Here's how the part is built. I have some questions about the finished solid (model axes, mm). Face numbers are marked on the shaded views. A direction names the side the tool comes from. Round coordinates to 2 decimals unless told otherwise and drop trailing zeros. Loops run counter-clockwise (first coordinate to the right, second up) from the corner with the lowest first, then second, coordinate; pieces in that order, holes last. Notation, with made-up numbers: M 37,31 L 70,31 A18 ccw 70,48 Z; hole C -5.5,79 d3. An arc over 180 degrees is marked long. Use a Markdown table: item, result.
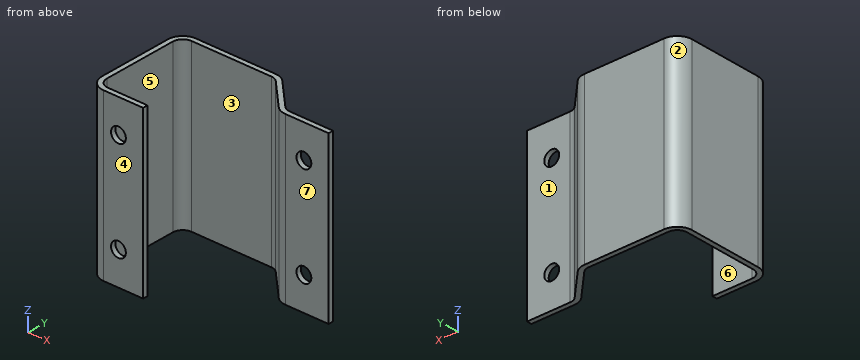
```python
from build123d import *

# Parameters (mm, degrees)
SKETCH1_W                    = 15
SKETCH1_H                    = 50
SKETCH1_R                    = 2.25
BASE_FLANGE1_DEPTH           = 1.5
EDGE_FLANGE1_STRIP_W         = 12
EDGE_FLANGE1_STRIP_H         = 1.5
EDGE_FLANGE1_STRIP_CUT_DEPTH = 50
EDGE_FLANGE1_DEPTH           = 50
EDGE_FLANGE2_STRIP_W         = 12
EDGE_FLANGE2_STRIP_H         = 1.5
EDGE_FLANGE2_STRIP_CUT_DEPTH = 50
EDGE_FLANGE2_DEPTH           = 50
EDGE_FLANGE3_STRIP_CUT_DEPTH = 50
EDGE_FLANGE3_DEPTH           = 50
EDGE_FLANGE4_STRIP_CUT_DEPTH = 50
EDGE_FLANGE4_DEPTH           = 50
SKETCH19_R                   = 2.25
CUT_EXTRUDE1_DEPTH           = 57.865713883


# Sheet-metal steps are written as plain solids
with BuildPart() as part:
    # Sketch1 → Base-Flange1 (new body)
    with BuildSketch(Plane(origin=(0, 0, 0), x_dir=(1, 0, 0), z_dir=(0, 1, 0))):
        Rectangle(SKETCH1_W, SKETCH1_H)
        with Locations(Location((0, 15, 0), (0, 0, 270))):
            Circle(SKETCH1_R, mode=Mode.SUBTRACT)
        with Locations(Location((0, -15, 0), (0, 0, 270))):
            Circle(SKETCH1_R, mode=Mode.SUBTRACT)
    extrude(amount=BASE_FLANGE1_DEPTH)

    # Edge-Flange1 strip (across the edge) → Edge-Flange1 strip cut (cut)
    with BuildSketch(Plane(origin=(-7.5, 1.5, -25), x_dir=(1, 0, 0), z_dir=(0, 0, 1))):
        with Locations((-3, -0.75)):
            Rectangle(EDGE_FLANGE1_STRIP_W, EDGE_FLANGE1_STRIP_H)
    extrude(amount=EDGE_FLANGE1_STRIP_CUT_DEPTH, mode=Mode.SUBTRACT)

    # Edge-Flange1 section (across the edge) → Edge-Flange1 (add)
    with BuildSketch(Plane(origin=(-7.5, 1.5, -25), x_dir=(1, 0, 0), z_dir=(0, 0, 1))):
        with BuildLine():
            Line((-1.5, 3), (-1.5, 28.5))
            Line((-1.5, 28.5), (0, 28.5))
            Line((0, 28.5), (0, 3))
            ThreePointArc((0, 3), (0.878679656, 0.878679656), (3, 0))
            Line((3, 0), (3, -1.5))
            ThreePointArc((3, -1.5), (-0.181980515, -0.181980515), (-1.5, 3))
        make_face()
    extrude(amount=EDGE_FLANGE1_DEPTH)

    # Edge-Flange2 strip (across the edge) → Edge-Flange2 strip cut (cut)
    with BuildSketch(Plane(origin=(-7.5, 30, -25), x_dir=(0, -1, 0), z_dir=(0, 0, 1))):
        with Locations((-3, -0.75)):
            Rectangle(EDGE_FLANGE2_STRIP_W, EDGE_FLANGE2_STRIP_H)
    extrude(amount=EDGE_FLANGE2_STRIP_CUT_DEPTH, mode=Mode.SUBTRACT)

    # Edge-Flange2 section (across the edge) → Edge-Flange2 (add)
    with BuildSketch(Plane(origin=(-7.5, 30, -25), x_dir=(0, -1, 0), z_dir=(0, 0, 1))):
        with BuildLine():
            Line((-1.5, 3), (-1.5, 28.5))
            Line((-1.5, 28.5), (0, 28.5))
            Line((0, 28.5), (0, 3))
            ThreePointArc((0, 3), (0.878679656, 0.878679656), (3, 0))
            Line((3, 0), (3, -1.5))
            ThreePointArc((3, -1.5), (-0.181980515, -0.181980515), (-1.5, 3))
        make_face()
    extrude(amount=EDGE_FLANGE2_DEPTH)

    # Edge-Flange3 strip (across the edge) → Edge-Flange3 strip cut (cut)
    with BuildSketch(Plane(origin=(21, 30, -25), x_dir=(-0.7071067811865389, -0.7071067811865561, 0), z_dir=(0, 0, 1))):
        Polygon((-8.66726189, 6.545941546), (-0.181980515, -1.939339828), (0.878679656, -0.878679656), (-7.606601718, 7.606601718), align=None)
    extrude(amount=EDGE_FLANGE3_STRIP_CUT_DEPTH, mode=Mode.SUBTRACT)

    # Edge-Flange3 section (across the edge) → Edge-Flange3 (add)
    with BuildSketch(Plane(origin=(21, 30, -25), x_dir=(-0.7071067811865389, -0.7071067811865561, 0), z_dir=(0, 0, 1))):
        with BuildLine():
            Line((-1.5, 1.242640687), (-1.5, 14.378679656))
            Line((-1.5, 14.378679656), (0, 14.378679656))
            Line((0, 14.378679656), (0, 1.242640687))
            ThreePointArc((0, 1.242640687), (0.228361402, 0.09459039), (0.878679656, -0.878679656))
            Line((0.878679656, -0.878679656), (-0.181980515, -1.939339828))
            ThreePointArc((-0.181980515, -1.939339828), (-1.157457896, -0.479434759), (-1.5, 1.242640687))
        make_face()
    extrude(amount=EDGE_FLANGE3_DEPTH)

    # Edge-Flange4 strip (across the edge) → Edge-Flange4 strip cut (cut)
    with BuildSketch(Plane(origin=(32.227922061, 20.893398282, 25), x_dir=(0, 1, 0), z_dir=(0, 0, -1))):
        Polygon((-8.66726189, 6.545941546), (-0.181980515, -1.939339828), (0.878679656, -0.878679656), (-7.606601718, 7.606601718), align=None)
    extrude(amount=EDGE_FLANGE4_STRIP_CUT_DEPTH, mode=Mode.SUBTRACT)

    # Edge-Flange4 section (across the edge) → Edge-Flange4 (add)
    with BuildSketch(Plane(origin=(32.227922061, 20.893398282, 25), x_dir=(0, 1, 0), z_dir=(0, 0, -1))):
        with BuildLine():
            Line((-1.5, 1.242640687), (-1.5, 14.378679656))
            Line((-1.5, 14.378679656), (0, 14.378679656))
            Line((0, 14.378679656), (0, 1.242640687))
            ThreePointArc((0, 1.242640687), (0.228361402, 0.09459039), (0.878679656, -0.878679656))
            Line((0.878679656, -0.878679656), (-0.181980515, -1.939339828))
            ThreePointArc((-0.181980515, -1.939339828), (-1.157457896, -0.479434759), (-1.5, 1.242640687))
        make_face()
    extrude(amount=EDGE_FLANGE4_DEPTH)

    # Sketch19 → Cut-Extrude1 (cut, through all)
    with BuildSketch(Plane(origin=(0, 20.893398282, 0), x_dir=(1, 0, 0), z_dir=(0, 1, 0))):
        with Locations(Location((39.106601718, 15, 0), (0, 0, 180))):
            Circle(SKETCH19_R)
        with Locations(Location((39.106601718, -15, 0), (0, 0, 180))):
            Circle(SKETCH19_R)
    extrude(amount=-CUT_EXTRUDE1_DEPTH, mode=Mode.SUBTRACT)


solid = part.part
```
Q1. We'd pull the mould along X, two halves only. Please class the marked faces 1, 2 and 3: pulls with the +X half, pulls with the -X half, needs draft (parallel to the pull), parting line crosses it, or undercut.
Return value:
| item | result |
|---|---|
| face 1 | needs draft |
| face 2 | pulls with the -X half |
| face 3 | undercut |
Q2. Will these pins go through, and if not, where does the flat tip stop? P1, Ø1.6, axis at y = 1, z = -3.5, coming from the +X side; P2, Ø8, axis at y = 28, z = 3.5, coming from the -X side; P3, Ø6, axis at x = 39.11, z = -15, coming from the +Y side; P4, Ø6, axis at x = 39.11, z = 15, coming from the -Y side.
Return value:
| item | result |
|---|---|
| P1 | stops at x = 7.5 |
| P2 | stops at x = -9 |
| P3 | stops at y = 20.89 |
| P4 | stops at y = 19.39 |
Q3. Imagine slicing it at A-A, the plane x = 3. Please give me the cut outline in (y, z), then the cut area to 3 significant figures.
Return value:
| item | result |
|---|---|
| outline | M 0,-25 L 1.5,-25 L 1.5,25 L 0,25 Z; M 30,-25 L 31.5,-25 L 31.5,25 L 30,25 Z |
| area | 150 mm^2 |
Q4. Imagine slicing it at C-C, the plane z = 7. Please give me the cut outline in (x, y).
Return value:
| item | result |
|---|---|
| outline | M -9,4.5 A4.5 ccw -4.5,0 L 7.5,0 L 7.5,1.5 L -4.5,1.5 A3 cw -7.5,4.5 L -7.5,27 A3 cw -4.5,30 L 19.76,30 A3 cw 21.88,29.12 L 30.29,20.71 A4.5 ccw 33.47,19.39 L 46.61,19.39 L 46.61,20.89 L 33.47,20.89 A3 cw 31.35,21.77 L 22.94,30.18 A4.5 ccw 19.76,31.5 L -4.5,31.5 A4.5 ccw -9,27 Z |
Q5. Imagine slicing it at D-D, the plane y = 26. Please give me the cut outline in (x, z), then the cut area to 3 significant figures.
Return value:
| item | result |
|---|---|
| outline | M -9,-25 L -7.5,-25 L -7.5,25 L -9,25 Z; M 25,-25 L 27.12,-25 L 27.12,25 L 25,25 Z |
| area | 181 mm^2 |
Q6. I need wall thicknesses on line 1 (X direction, y = 20, z = 14); line 2 (Y direction, x = 7, z = 23); line 3 (X direction, y = 5.5, z = -4). Which ranges of each line are inside material? Lowest first, please. Write a range as from..to.
Return value:
| item | result |
|---|---|
| line 1 | x = -9..-7.5, 31.21..37.09, 41.12..46.61 |
| line 2 | y = 0..1.5, 30..31.5 |
| line 3 | x = -9..-7.5 |
Q7. Imagine slicing it at B-B, the plane z = -15. Please give me the cut outline in (x, y).
Return value:
| item | result |
|---|---|
| outline | M -9,4.5 A4.5 ccw -4.5,0 L -2.25,0 L -2.25,1.5 L -4.5,1.5 A3 cw -7.5,4.5 L -7.5,27 A3 cw -4.5,30 L 19.76,30 A3 cw 21.88,29.12 L 30.29,20.71 A4.5 ccw 33.47,19.39 L 36.86,19.39 L 36.86,20.89 L 33.47,20.89 A3 cw 31.35,21.77 L 22.94,30.18 A4.5 ccw 19.76,31.5 L -4.5,31.5 A4.5 ccw -9,27 Z; M 2.25,0 L 7.5,0 L 7.5,1.5 L 2.25,1.5 Z; M 41.36,19.39 L 46.61,19.39 L 46.61,20.89 L 41.36,20.89 Z |
Q8. For the marked faces 4, 5, 6 and 7, which set-ups out of +Z, -Z, +X, -X, +Y, -Y let a thin tool reach every point of the face, with its end or its side?
Return value:
| item | result |
|---|---|
| face 4 | +Z, -Z, +X, -X, -Y |
| face 5 | +Z, -Z |
| face 6 | +Z, -Z, +X |
| face 7 | +Z, -Z, +X, -Y |
